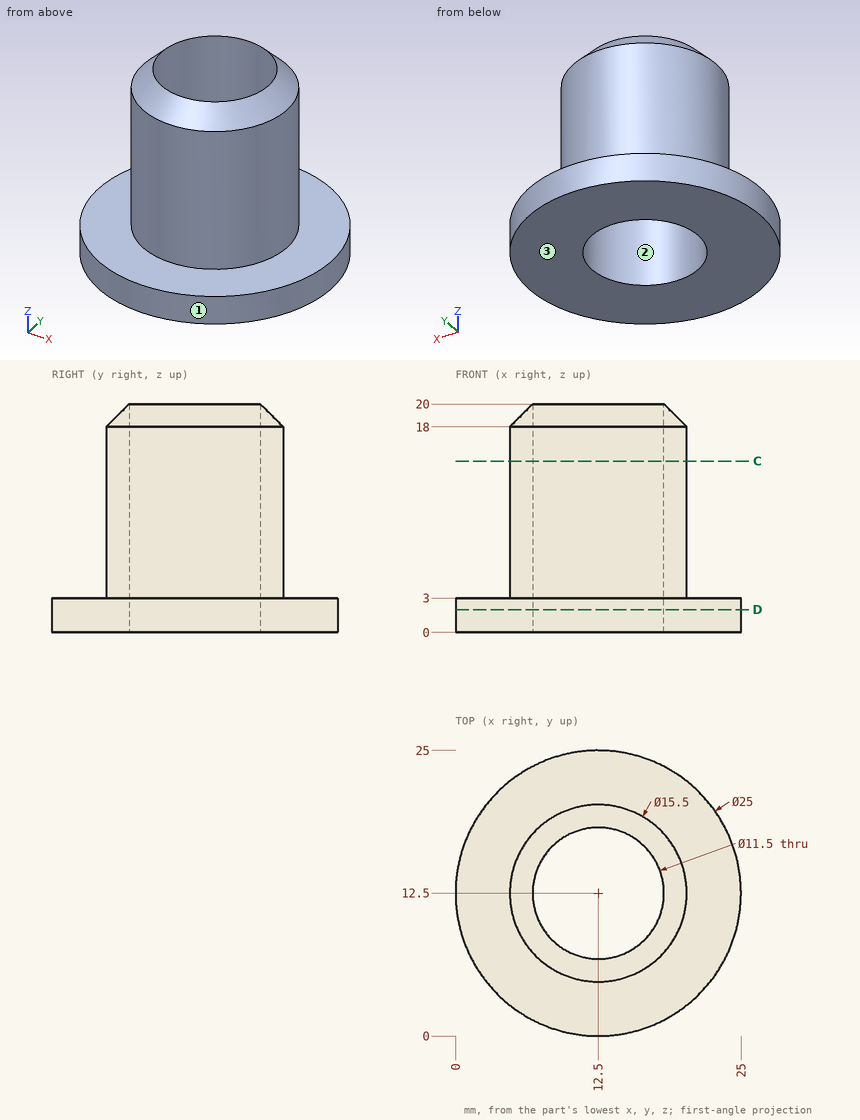
Verification items for this drawing (mm, ordinates from the low corner). Give positions to 0.01 mm unless a question says otherwise; leave off trailing zeros. Loops run counter-clockwise (first coordinate to the right, second up) from the corner with the lowest first, then second, coordinate; pieces in that order, holes last. Notation, with made-up numbers: M 49,35 L 65,35 A27 ccw 65,55 Z; hole C 72,-15.75 d5. An arc over 180 degrees is marked long. Answer as a JSON object with one key per item and string values. Group by question number.
Item 1: Mould release check, pull along X, two halves, no side actions. Record for the marked faces 1, 2 and 3: pulls with the +X half, pulls with the -X half, needs draft (parallel to the pull), parting line crosses it, or undercut.
Item 2: Sectioned sample at C-C on z = 15. Record the boundary of the cut face in (x, y).
Item 3: Material ranges on L1, parallel to Y at x = 12.5, z = 9.5; L2, parallel to Z at x = 5.5, y = 6.25; L3, parallel to X at y = 7.25, z = 13.75, recorded low to high.
Item 4: Sectioned sample at D-D on z = 2. Record the boundary of the cut face in (x, y).
Item 5: Gauge pin test, flat ends, axial feed: pin 1 (4 mm diameter, centred on y = 21.5, z = 4.5, fed in from +X); pin 2 (1 mm diameter, centred on y = 16.5, z = 15.5, fed in from -X); pin 3 (1 mm diameter, centred on x = 11.5, z = 16, fed in from +Y). Record the tip position at first contact, or that the pin passes through.
Findings below:
{
 "1": {"face 1": "parting line crosses it", "face 2": "undercut", "face 3": "needs draft"},
 "2": {"outline": "C 12.5,12.5 d15.5; hole C 12.5,12.5 d11.5"},
 "3": {"L1": "4.75 to 6.75, 18.25 to 20.25", "L2": "0 to 3", "L3": "6.8 to 10.15, 14.85 to 18.2"},
 "4": {"outline": "C 12.5,12.5 d25; hole C 12.5,12.5 d11.5"},
 "5": {"pin 1": "x = 22.36", "pin 2": "x = 5.59", "pin 3": "y = 20.23"}
}
